Check sheet for the modelled part. Datum: model origin and axes. Units: mm. Coordinates: 2 decimals unless noted, no trailing zeros. Loops run counter-clockwise (first coordinate to the right, second up) from the corner with the lowest first, then second, coordinate; pieces in that order, holes last.
```python
from build123d import *

# Parameters (mm, degrees)
SKETCH1_R           = 2.1828125
BOSS_EXTRUDE1_DEPTH = 0.79375


with BuildPart() as part:
    # Sketch1 → Boss-Extrude1 (new, symmetric)
    with BuildSketch(Plane(origin=(0, 0, 0), x_dir=(1, 0, 0), z_dir=(0, 1, 0))):
        with BuildLine():
            Line((-6.35, 0), (-6.35, 50.8))
            ThreePointArc((-6.35, 50.8), (-4.490128061, 55.290128061), (0, 57.15))
            Line((0, 57.15), (3.719743879, 57.15))
            ThreePointArc((3.719743879, 57.15), (6.149783674, 56.666635031), (8.209871939, 55.290128061))
            Line((8.209871939, 55.290128061), (55.290128061, 8.209871939))
            ThreePointArc((55.290128061, 8.209871939), (56.666635031, 6.149783674), (57.15, 3.719743879))
            Line((57.15, 3.719743879), (57.15, 0))
            ThreePointArc((57.15, 0), (55.290128061, -4.490128061), (50.8, -6.35))
            Line((50.8, -6.35), (0, -6.35))
            ThreePointArc((0, -6.35), (-4.490128061, -4.490128061), (-6.35, 0))
        make_face()
        with Locations(Location((0, 0, 0), (0, 0, 270))):
            Circle(SKETCH1_R, mode=Mode.SUBTRACT)
        with Locations(Location((0, 50.8, 0), (0, 0, 270))):
            Circle(SKETCH1_R, mode=Mode.SUBTRACT)
        with Locations(Location((50.8, 0, 0), (0, 0, 270))):
            Circle(SKETCH1_R, mode=Mode.SUBTRACT)
        with Locations(Location((25.4, 0, 0), (0, 0, 270))):
            Circle(SKETCH1_R, mode=Mode.SUBTRACT)
        with Locations(Location((0, 38.1, 0), (0, 0, 270))):
            Circle(SKETCH1_R, mode=Mode.SUBTRACT)
        with Locations(Location((25.4, 25.4, 0), (0, 0, 270))):
            Circle(SKETCH1_R, mode=Mode.SUBTRACT)
    extrude(amount=BOSS_EXTRUDE1_DEPTH, both=True)


solid = part.part
```
1) Mould release check, pull along Z, two halves, no side actions. Record for faces 1 (the flat face through (26, 0, 6.35)), 2 (the cylindrical face through (0.1, -0.01, -52.98)), 3 (the flat face through (2, 0, -57.15)): +Z half, -Z half, draft (parallel to the pull), parting line (faces both ways), or undercut.
Answer sheet:
face 1: +Z half
face 2: undercut
face 3: -Z half
2) Section check B-B on z = -38.1. Enter the section's corners in (x, y), plus the area to 3 significant figures.
Answer sheet:
outline: (-6.35, -0.79) - (-2.18, -0.79) - (-2.18, 0.79) - (-6.35, 0.79) - close; (2.18, -0.79) - (25.4, -0.79) - (25.4, 0.79) - (2.18, 0.79) - close
area: 43.5 mm2
3) Section check C-C on y = 0.15. Enter the section's corners in (x, z), plus the area to 3 significant figures.
Answer sheet:
outline: (-6.35, -50.8) arc R6.35 ccw to (0, -57.15) - (3.72, -57.15) arc R6.35 ccw to (8.21, -55.29) - (55.29, -8.21) arc R6.35 ccw to (57.15, -3.72) - (57.15, 0) arc R6.35 ccw to (50.8, 6.35) - (0, 6.35) arc R6.35 ccw to (-6.35, 0) - close; hole circle Ø4.37 at (0, -50.8); hole circle Ø4.37 at (0, -38.1); hole circle Ø4.37 at (0, 0); hole circle Ø4.37 at (25.4, -25.4); hole circle Ø4.37 at (25.4, 0); hole circle Ø4.37 at (50.8, 0)
area: 2,620 mm2
4) Section check A-A on x = 25.4. Enter the section's corners in (y, z).
Answer sheet:
outline: (-0.79, -38.1) - (0.79, -38.1) - (0.79, -27.58) - (-0.79, -27.58) - close; (-0.79, -23.22) - (0.79, -23.22) - (0.79, -2.18) - (-0.79, -2.18) - close; (-0.79, 2.18) - (0.79, 2.18) - (0.79, 6.35) - (-0.79, 6.35) - close
5) Section check D-D on z = -25.4. Enter the section's corners in (x, y), plus the area to 3 significant figures.
Answer sheet:
outline: (-6.35, -0.79) - (23.22, -0.79) - (23.22, 0.79) - (-6.35, 0.79) - close; (27.58, -0.79) - (38.1, -0.79) - (38.1, 0.79) - (27.58, 0.79) - close
area: 63.6 mm2
6) Scan lines: line 1 (Z direction, x = 1.5, y = -0.6); line 2 (Z direction, x = 24, y = -0.55); line 3 (Z direction, x = 23.5, y = 0.2). Record each from-to range of solid material in increasing order.
Answer sheet:
line 1: z = -57.15 to -52.39, -49.21 to -39.69, -36.51 to -1.59, 1.59 to 6.35
line 2: z = -39.5 to -27.07, -23.73 to -1.67, 1.67 to 6.35
line 3: z = -40 to -26.47, -24.33 to -1.07, 1.07 to 6.35
